Answer from the drawing. Dimensions are ordinates in mm from the lowest x, y and z of the part. A direction names the side the tool comes from. Give positions to 0.01 mm unless a question says otherwise; leave off trailing zeros. Loops run counter-clockwise (first coordinate to the right, second up) from the corner with the lowest first, then second, coordinate; pieces in that order, holes last. Notation, with made-up numbers: M -27.75,-28 L 4.25,-28 A5 cw 4.25,-23 Z; hole C 81,87.5 d9. An arc over 180 degrees is marked long. Return JSON: item names as keys, results as strings. Group by question number.
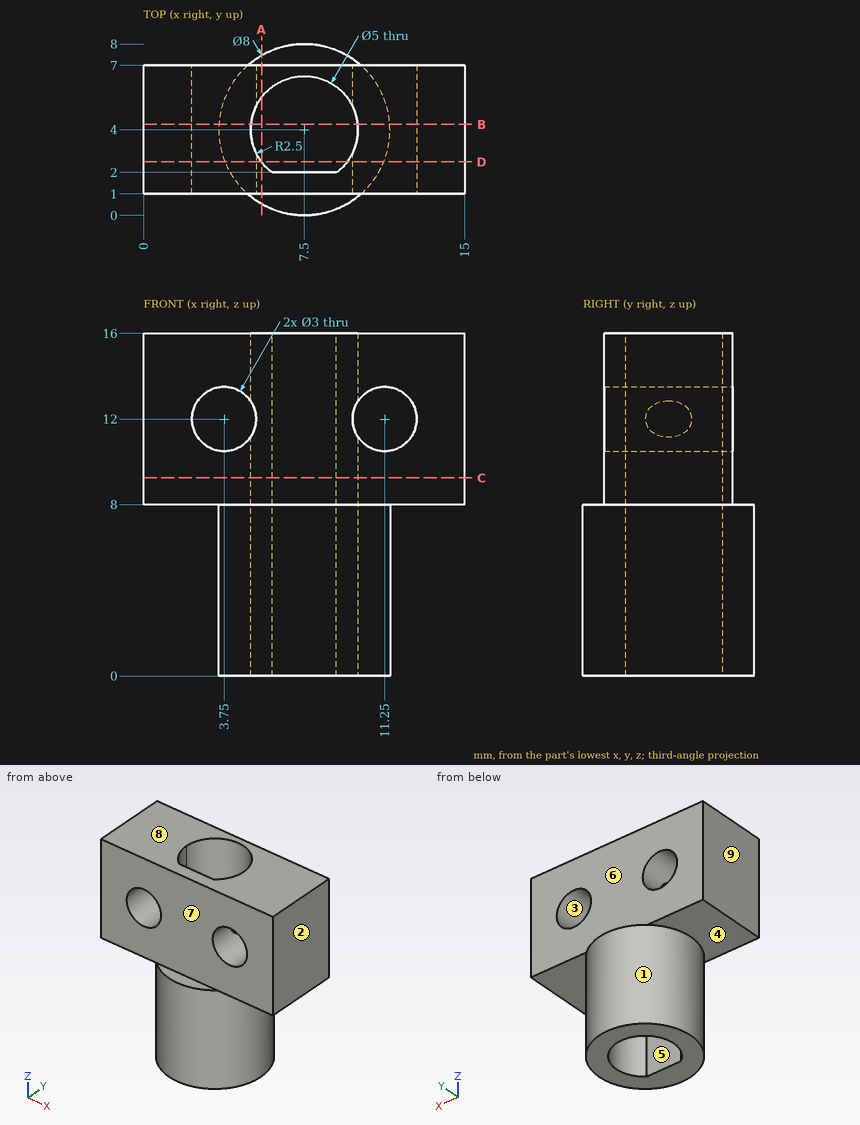
1. Find section D-D (y = 2.5). Write down the section's boundary in (x, z).
2. Find section A-A (x = 5.5). Write down the section's boundary in (y, z).
3. Flat-ended cylindrical pins translate along their axes: P1, Ø5, axis at x = 11.25, z = 12, coming from the +Y side; P2, Ø0.8, axis at x = 7.5, y = 0.5, coming from the +Z side; P3, Ø1.5, axis at y = 1, z = 3.5, coming from the -X side. Find the tip coordinate at first contact, or state that the pin passes through.
4. Straight lines are drawn through the part: line 1 along Y through (x, z) = (7.5, 9.75); line 2 along X through (y, z) = (4, 3.75); line 3 along Y through (x, z) = (7.5, 4.25). For each, find the intervals that lie inside material, in ascending order.
5. Find section C-C (z = 9.25). Write down the section's boundary in (x, y).
6. For the marked faces 5, 6, 7, 8 and 9, determine the directions among +Z, -Z, +X, -X, +Y, -Y from which every point of the face is accessible in a straight line to the end or side of a thin tool.
7. Find section B-B (y = 4.25). Write down the section's boundary in (x, z), and give its area (3 significant figures).
8. The mould has two halves that part along X. Classify the marked faces 1, 2, 3 and 4: +X half, -X half, draft (parallel to the pull), parting line (faces both ways), or undercut.
Result:
{
 "1": {"outline": "M 0,8 L 3.79,8 L 3.79,0 L 5.5,0 L 5.5,16 L 0,16 Z; M 9.5,0 L 11.21,0 L 11.21,8 L 15,8 L 15,16 L 9.5,16 Z; hole C 3.75,12 d3; hole C 11.25,12 d3"},
 "2": {"outline": "M 0.54,0 L 2.5,0 L 2.5,16 L 1,16 L 1,8 L 0.54,8 Z; M 5.5,0 L 7.46,0 L 7.46,8 L 7,8 L 7,16 L 5.5,16 Z"},
 "3": {"P1": "stops at y = 7", "P2": "stops at z = 8", "P3": "stops at x = 4.19"},
 "4": {"line 1": "y = 1 to 2, 6.5 to 7", "line 2": "x = 3.5 to 5, 10 to 11.5", "line 3": "y = 0 to 2, 6.5 to 8"},
 "5": {"outline": "M 0,1 L 15,1 L 15,7 L 0,7 Z; hole M 6,2 L 9,2 A2.5 ccw long Z"},
 "6": {"face 5": "+Z, -Z", "face 6": "+Z, +X, -X, +Y", "face 7": "+Z, +X, -X, -Y", "face 8": "+Z, +X, -X, +Y, -Y", "face 9": "+Z, -Z, -X, +Y, -Y"},
 "7": {"outline": "M 0,8 L 3.51,8 L 3.51,0 L 5.01,0 L 5.01,11.19 A1.5 cw long 5.01,12.81 L 5.01,16 L 0,16 Z; M 9.99,0 L 11.49,0 L 11.49,8 L 15,8 L 15,16 L 9.99,16 L 9.99,12.81 A1.5 cw long 9.99,11.19 Z", "area": "90.7 mm2"},
 "8": {"face 1": "parting line", "face 2": "+X half", "face 3": "undercut", "face 4": "draft"}
}
